Part model, mm, in its own coordinate system. A direction names the side the tool comes from. Give positions to 0.01 mm unless a question says otherwise; leave off trailing zeros. Order: outer loops, then holes, each group sorted by start corner. A loop starts at its lowest first (then second) coordinate and runs counter-clockwise, first axis right, second up.
from build123d import *

# Parameters (mm, degrees)
EXTRUDE_2_DEPTH         = 8
SKETCH_1_11_OUTSIDE_W   = 54.492
SKETCH_1_11_OUTSIDE_H   = 61.792
SKETCH_1_11_OUTSIDE_R   = 6
SKETCH_1_11_OUTSIDE_R_2 = 1.5
CUT_EXTRUDE_2_DEPTH     = 63.460307396
EXTRUDE_4_DEPTH         = 40
SKETCH_9_R              = 1.5
CUT_EXTRUDE_3_DEPTH     = 66.295934524
FILLET_1_R              = 5
FILLET_2_R              = 5


with BuildPart() as part:
    # Эскиз1 → Бобышка-Вытянуть2 (new body)
    with BuildSketch(Plane.XY):
        with BuildLine():
            Line((0, 0), (40, 0))
            Line((40, 0), (40, 27.3))
            ThreePointArc((40, 27.3), (20, 47.3), (0, 27.3))
            Line((0, 27.3), (0, 0))
        make_face()
    extrude(amount=EXTRUDE_2_DEPTH)

    # Эскиз1<11> outside → Вырез-Вытянуть2 (cut, through all)
    # profile 1 of 8: a face of its own
    with BuildSketch(Plane.XY):
        with Locations((20, 23.65)):
            Rectangle(SKETCH_1_11_OUTSIDE_W, SKETCH_1_11_OUTSIDE_H)
        with BuildLine():
            Line((0, 0), (40, 0))
            Line((40, 0), (40, 27.3))
            ThreePointArc((40, 27.3), (20, 47.3), (0, 27.3))
            Line((0, 27.3), (0, 0))
        make_face(mode=Mode.SUBTRACT)
    # profile 2 of 8: a face of its own
    with BuildSketch(Plane.XY):
        with Locations((20, 20)):
            Circle(SKETCH_1_11_OUTSIDE_R)
    # profile 3 of 8: a face of its own
    with BuildSketch(Plane.XY):
        with Locations((3.37, 27.3)):
            Circle(SKETCH_1_11_OUTSIDE_R_2)
    # profile 4 of 8: a face of its own
    with BuildSketch(Plane.XY):
        with Locations((11.685, 41.702002465)):
            Circle(SKETCH_1_11_OUTSIDE_R_2)
    # profile 5 of 8: a face of its own
    with BuildSketch(Plane.XY):
        with Locations((28.315, 41.702002465)):
            Circle(SKETCH_1_11_OUTSIDE_R_2)
    # profile 6 of 8: a face of its own
    with BuildSketch(Plane.XY):
        with Locations((36.63, 27.3)):
            Circle(SKETCH_1_11_OUTSIDE_R_2)
    # profile 7 of 8: a face of its own
    with BuildSketch(Plane.XY):
        with Locations((28.315, 12.897997535)):
            Circle(SKETCH_1_11_OUTSIDE_R_2)
    # profile 8 of 8: a face of its own
    with BuildSketch(Plane.XY):
        with Locations((11.685, 12.897997535)):
            Circle(SKETCH_1_11_OUTSIDE_R_2)
    extrude(amount=CUT_EXTRUDE_2_DEPTH, mode=Mode.SUBTRACT)

    # Эскиз8 → Бобышка-Вытянуть4 (add)
    with BuildSketch(Plane(origin=(0, 0, 0), x_dir=(-1, 0, 0), z_dir=(0, 0, -1))):
        with BuildLine():
            Line((-33.397427614, 14.687746699), (-40, 14.687746699))
            Line((-40, 14.687746699), (-40, 0))
            Line((-40, 0), (0, 0))
            Line((0, 0), (0, 14.687746699))
            Line((0, 14.687746699), (-6.602572386, 14.687746699))
            ThreePointArc((-6.602572386, 14.687746699), (-20, 8.9), (-33.397427614, 14.687746699))
        make_face()
    extrude(amount=EXTRUDE_4_DEPTH)

    # Эскиз9 → Вырез-Вытянуть3 (cut, through all)
    with BuildSketch(Plane(origin=(0, 14.687746699, 0), x_dir=(1, 0, 0), z_dir=(0, 1, 0))):
        with Locations(Location((36.487813402, 5.586160045, 0), (0, 0, 270))):
            Circle(SKETCH_9_R)
        with Locations(Location((3.174622012, 5.586160045, 0), (0, 0, 270))):
            Circle(SKETCH_9_R)
        with Locations(Location((3.174622012, 30.147789022, 0), (0, 0, 270))):
            Circle(SKETCH_9_R)
        with Locations(Location((36.487813402, 30.147789022, 0), (0, 0, 270))):
            Circle(SKETCH_9_R)
    extrude(amount=-CUT_EXTRUDE_3_DEPTH, mode=Mode.SUBTRACT)

    # Скругление1
    # the kernel refuses this fillet: 5 mm, written as the material it adds along each edge
    with BuildSketch(Plane(origin=(20.897427614, 14.687746699, 0), x_dir=(0, 1, 0), z_dir=(1, 0, 0))) as fillet_1_piece_1_section:
        with BuildLine():
            CenterArc((FILLET_1_R, -FILLET_1_R), FILLET_1_R, 90, 90)
            Line((0, -FILLET_1_R), (0, 0))
            Line((0, 0), (FILLET_1_R, 0))
        make_face()
    fillet_1_piece_1 = extrude(amount=19.102572386, mode=Mode.PRIVATE)
    fillet_1_piece_1 = fillet_1_piece_1 - Plane(origin=(20, 27.3, -1.204390543), x_dir=(-0.7281210659848666, -0.6854485489583165, 0), z_dir=(0, 0, 1)) * Cylinder(18.4, 59, mode=Mode.PRIVATE)
    fillet_1_piece_1 = fillet_1_piece_1 - Plane(origin=(36.487813402, 15.674506784, -5.586160045), x_dir=(0, 0, 1), z_dir=(0, 1, 0)) * Cylinder(1.5, 59, mode=Mode.PRIVATE)
    add(fillet_1_piece_1)

    # Скругление2
    # the kernel refuses this fillet: 5 mm, written as the material it adds along each edge
    with BuildSketch(Plane(origin=(0, 14.687746699, 0), x_dir=(0, 0, -1), z_dir=(1, 0, 0))) as fillet_2_piece_1_section:
        with BuildLine():
            CenterArc((FILLET_2_R, FILLET_2_R), FILLET_2_R, 180, 90)
            Line((0, FILLET_2_R), (0, 0))
            Line((0, 0), (FILLET_2_R, 0))
        make_face()
    fillet_2_piece_1 = extrude(amount=19.102572386, mode=Mode.PRIVATE)
    fillet_2_piece_1 = fillet_2_piece_1 - Plane(origin=(20, 27.3, -1.204389903), x_dir=(-0.7281210659850873, -0.6854485489580822, 0), z_dir=(0, 0, 1)) * Cylinder(18.4, 59, mode=Mode.PRIVATE)
    fillet_2_piece_1 = fillet_2_piece_1 - Plane(origin=(3.174622012, 15.67450541, -5.586160045), x_dir=(0, 0, 1), z_dir=(0, 1, 0)) * Cylinder(1.5, 59, mode=Mode.PRIVATE)
    add(fillet_2_piece_1)


solid = part.part
Item 1: Drill centre lines: probe 1 along X at (y, z) = (27.3, 3.25); probe 2 along Z at (x, y) = (4, 4); probe 3 along Y at (x, z) = (20, 2). Where is each one in solid material? Low to high.
Item 2: Pull direction Z, two halves, no side cores. Call faces 4 (the face through (2.521, 16.191, -1.426)), 5 (the face through (4.176, 28.565, 3.944)), 6 (the face through (35.157, 7.447, -29.456)): released by +Z, released by -Z, zero draft, split by the parting line, or undercut.
Item 3: Band-saw the part on B-B on y = 25. List the corners of the cut face in (x, z).
Item 4: Band-saw the part on D-D on x = 31. List the corners of the cut face in (y, z), plus the area to 3 significant figures.
Item 5: Band-saw the part on A-A on x = 20. List the corners of the cut face in (y, z), plus the area to 3 significant figures.
Item 6: Drop flat-ended pins along their axis: P1, Ø6, axis at x = 33, z = -7, coming from the -Y side; P2, Ø8, axis at x = 13, z = -28.5, coming from the +Y side; P3, Ø10, axis at y = 23.5, z = -27, coming from the +X side; P4, Ø2, axis at x = 4.5, z = -26, coming from the +Y side. Give the stop position or say it passes through.
Item 7: Which spindle directions (+Z, -Z, +X, -X, +Y, -Y) get a long thin tool onto all of the face, cutting with end or side? Do faces 1 (the face through (0, 8, -16)), 2 (the face through (37, 14.688, -22)), 3 (the face through (20, 28, 0)). Say none if no direction does.
Item 8: Band-saw the part on C-C on z = 3. List the corners of the cut face in (x, y) (3 decimals).
Working result:
1. probe 1: x = 0 to 1.87, 4.87 to 35.13, 38.13 to 40
1. probe 2: z = -40 to -31.4, -28.9 to -6.84, -4.33 to 8
1. probe 3: y = 0 to 14, 26 to 47.3
2. face 4: released by -Z
2. face 5: zero draft
2. face 6: undercut
3. outline: (0, 0) - (16.68, 0) - (16.68, 8) - (0, 8) - close; (23.32, 0) - (40, 0) - (40, 8) - (23.32, 8) - close
4. outline: (0, -40) - (12.55, -40) - (12.55, 0) - (44, 0) - (44, 8) - (0, 8) - close
4. area: 854 mm2
5. outline: (0, -40) - (8.9, -40) - (8.9, 0) - (14, 0) - (14, 8) - (0, 8) - close; (26, 0) - (47.3, 0) - (47.3, 8) - (26, 8) - close
5. area: 638 mm2
6. P1: stops at y = 0
6. P2: stops at y = 12.55
6. P3: passes through
6. P4: stops at y = 14.69
7. face 1: +Z, -Z, -X, +Y, -Y
7. face 2: -Z, +X, -X, +Y
7. face 3: -Z, +Y
8. outline: (0, 0) - (40, 0) - (40, 27.3) arc R20 ccw to (0, 27.3) - close; hole circle Ø3 at (3.37, 27.3); hole circle Ø3 at (11.685, 12.898); hole circle Ø3 at (11.685, 41.702); hole circle Ø12 at (20, 20); hole circle Ø3 at (28.315, 12.898); hole circle Ø3 at (28.315, 41.702); hole circle Ø3 at (36.63, 27.3)
